Verification items for the finished model (mm, model axes). A direction names the side the tool comes from. Give positions to 0.01 mm unless a question says otherwise; leave off trailing zeros. Loops run counter-clockwise (first coordinate to the right, second up) from the corner with the lowest first, then second, coordinate; pieces in that order, holes last. Notation, with made-up numbers: M 18,60.5 L 38,60.5 A21 ccw 38,98.5 Z; hole C 75,-34.5 d8. An arc over 180 degrees is marked long. Answer in a Markdown table with one row per item.
```python
from build123d import *

# Parameters (mm, degrees)
F1_DEPTH = 1104
F2_W     = 193.684367
F2_H     = 94
F2_W_2   = 206.995809
F3_DEPTH = 19
F4_W     = 75
F4_H     = 19
F5_DEPTH = 19


with BuildPart() as f1:
    # F0 (on Front) → F1 (new body, symmetric)
    with BuildSketch(Plane.XZ):
        Polygon((0, -19), (0, 0), (-75, 0), (-75, -19), (-95, -19), (-95, -38), (-139, -38), (-139, -57), (-20, -57), (-20, -19), align=None)
    extrude(amount=F1_DEPTH, both=True)

    # F2 (on face) → F3 (cut)
    with BuildSketch(Plane(origin=(0, 0, -57), x_dir=(1, 0, 0), z_dir=(0, 0, -1))):
        with Locations((-42.157817, 1057)):
            Rectangle(F2_W, F2_H)
        with Locations((-35.502096, -1057)):
            Rectangle(F2_W_2, F2_H)
    extrude(amount=-F3_DEPTH, mode=Mode.SUBTRACT)

    # F4 (on face) → F5 (cut)
    with BuildSketch(Plane(origin=(0, 0, -38), x_dir=(1, 0, 0), z_dir=(0, 0, -1))):
        with Locations((-57.5, 1094.5)):
            Rectangle(F4_W, F4_H)
        with Locations((-57.5, -1094.5)):
            Rectangle(F4_W, F4_H)
    extrude(amount=-F5_DEPTH, mode=Mode.SUBTRACT)


solid = f1.part
```
Item 1: Go/stop test with flat-tipped pins: pin 1 (5.5 mm diameter, centred on y = -454.5, z = -8.5, fed in from -X); pin 2 (16 mm diameter, centred on x = -89, y = -114.5, fed in from +Z); pin 3 (15 mm diameter, centred on x = -95.5, z = -49.5, fed in from -Y). Record where each tip stops, or that it passes through.
Reported:
| item | result |
|---|---|
| pin 1 | stops at x = -75 |
| pin 2 | stops at z = -19 |
| pin 3 | stops at y = -1010 |
Item 2: Sectioned sample at D-D (x = -121). Record the cut outline in (y, z), and give its area (3 significant figures).
Reported:
| item | result |
|---|---|
| outline | M -1010,-57 L 1010,-57 L 1010,-38 L -1010,-38 Z |
| area | 38,400 mm^2 |
Item 3: Sectioned sample at C-C (z = -47). Record the cut outline in (x, y), and give its area (3 significant figures).
Reported:
| item | result |
|---|---|
| outline | M -139,-1010 L -20,-1010 L -20,1010 L -139,1010 Z |
| area | 240,000 mm^2 |
Item 4: Scan lines: L1, parallel to Z at x = -12, y = -453; L2, parallel to X at y = 772, z = -41.5; L3, parallel to Z at x = -99, y = -639. Record each from-to range of solid material in increasing order. Write a range as [from, to].
Reported:
| item | result |
|---|---|
| L1 | z = [-19, 0] |
| L2 | x = [-139, -20] |
| L3 | z = [-57, -38] |
Item 5: Sectioned sample at A-A (y = 659.5). Record the cut outline in (x, z), and give its area (3 significant figures).
Reported:
| item | result |
|---|---|
| outline | M -139,-57 L -20,-57 L -20,-19 L 0,-19 L 0,0 L -75,0 L -75,-19 L -95,-19 L -95,-38 L -139,-38 Z |
| area | 5,110 mm^2 |
Item 6: Sectioned sample at B-B (x = -38.5). Record the cut outline in (y, z).
Reported:
| item | result |
|---|---|
| outline | M -1104,-19 L -1085,-19 L -1085,-38 L -1010,-38 L -1010,-57 L 1010,-57 L 1010,-38 L 1085,-38 L 1085,-19 L 1104,-19 L 1104,0 L -1104,0 Z |
Item 7: Tool access check on faces 1 (the flat face through (-58, -1048, -38)), 2 (the flat face through (-37, -15, 0)), 3 (the flat face through (-20, -15, -38)), 4 (the flat face through (-117, -14, -38)), 5 (the flat face through (-58, 1047, -38)). Record the directions out of +Z, -Z, +X, -X, +Y, -Y that give a thin tool (end or side, any length) a straight path to the whole face; none if there is none.
Reported:
| item | result |
|---|---|
| face 1 | -Z, +X, -X, -Y |
| face 2 | +Z, +X, -X, +Y, -Y |
| face 3 | -Z, +X, +Y, -Y |
| face 4 | +Z, -X, +Y, -Y |
| face 5 | -Z, +X, -X, +Y |
